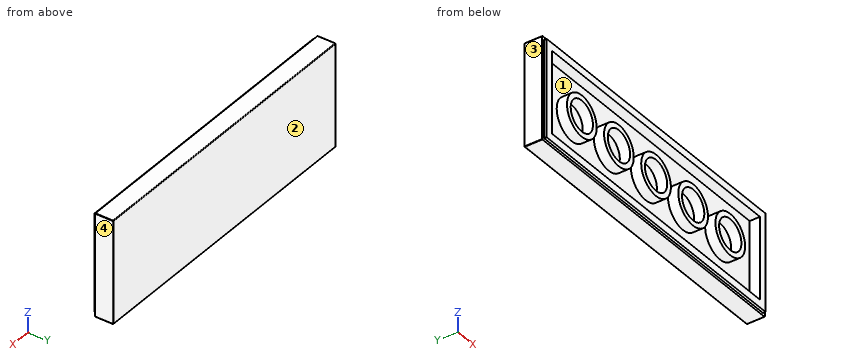
Autodesk Inventor part; units mm, degrees
ref_plane "YZ Plane" through (0, 0, 0) normal (1, 0, 0) x (0, 1, 0)
ref_plane "XZ Plane" through (0, 0, 0) normal (0, 1, 0) x (-1, 0, 0)
ref_plane "XY Plane" through (0, 0, 0) normal (0, 0, 1) x (1, 0, 0)
sketch "Sketch2" plane through (0, 0, 0) normal (0, 1, 0) x (-1, 0, 0)
  line L0 (-24, 8) -> (24, 8)
  line L1 (24, 8) -> (24, -8)
  line L2 (24, -8) -> (-24, -8)
  line L3 (-24, -8) -> (-24, 8)
  line L4 (-23.6, 7.6) -> (23.6, 7.6)
  line L5 (23.6, 7.6) -> (23.6, -7.6)
  line L6 (23.6, -7.6) -> (-23.6, -7.6)
  line L7 (-23.6, -7.6) -> (-23.6, 7.6)
  circle A0 centre (0, 0) radius 2.4
  circle A1 centre (0, 0) radius 3.2
  circle A2 centre (-8, 0) radius 2.4
  circle A3 centre (-8, 0) radius 3.2
  circle A4 centre (-16, 0) radius 2.4
  circle A5 centre (-16, 0) radius 3.2
  circle A6 centre (8, 0) radius 2.4
  circle A7 centre (8, 0) radius 3.2
  circle A8 centre (16, 0) radius 2.4
  circle A9 centre (16, 0) radius 3.2
  line L8 (16, 0) -> (8, 0) construction
  line L9 (8, 0) -> (0, 0) construction
  line L10 (0, 0) -> (-8, 0) construction
  line L11 (-8, 0) -> (-16, 0) construction
  line L12 (-22.4, 6.4) -> (22.4, 6.4)
  line L13 (22.4, 6.4) -> (22.4, -6.4)
  line L14 (22.4, -6.4) -> (-22.4, -6.4)
  line L15 (-22.4, -6.4) -> (-22.4, 6.4)
  circle A10 centre (-20, 4) radius 2.4 construction
  circle A11 centre (-20, -4) radius 2.4 construction
  circle A12 centre (20, 4) radius 2.4 construction
  circle A13 centre (20, -4) radius 2.4 construction
  point P0 (0, 8)
  point P1 (-24, 0)
  point P2 (0, 7.6)
  point P3 (-23.6, 0)
  point P4 (0, 6.4)
  point P5 (-22.4, 0)
  dimension "d0" = 16
  dimension "d1" = 48
  dimension "d2" = 0.4
  dimension "d3" = 0.4
  dimension "d4" = 4.8
  dimension "d5" = 6.4
  dimension "d6" = 8
  dimension "d7" = 1.6
  dimension "d8" = 1.6
  dimension "d15" = 4.8
extrude "Extrusion1" add sketch "Sketch2" along normal blind 3.2 contours L0 L1 L2 L3 | L4 L5 L6 L7 | A0 | A1 | A2 | A3 | A4 | A5 | A6 | A7 | A8 | A9 | L12 L13 L14 L15
extrude "Extrusion2" cut sketch "Sketch2" along normal blind 0.4 contours L0 L1 L2 L3
extrude "Extrusion3" cut sketch "Sketch2" along normal blind 1.6 contours A0 | A2 | A4 | A6 | A8 | L12 L13 L14 L15
fillet "Fillet1" radius 0.1 8 edges at (-24, 1.8, 8) (0, 3.2, 8) (-24, 3.2, 0) (-24, 1.8, -8) (0, 3.2, -8) (24, 1.8, -8) (24, 3.2, 0) (24, 1.8, 8)
sketch "Skizze3" plane through (0, 3.2, 0) normal (0, 1, 0) x (1, 0, 0)
  line L0 (23.9, 8) -> (-23.9, 8)
  line L1 (-24, 7.9) -> (-24, -7.9)
  line L2 (-23.9, -8) -> (23.9, -8)
  line L3 (23.9, -7.9) -> (-23.9, -7.9)
  line L4 (-24.9, -8.5) -> (-24.9, 8.1) construction
  line L5 (-24.9, 8.1) -> (28.7985, 8.1) construction
  line L6 (28.7985, 8.1) -> (28.7985, -8.5) construction
  line L7 (28.7985, -8.5) -> (-24.9, -8.5) construction
  point P0 (0, 0)
  dimension "d43" = 0.1
  dimension "d44" = 0.6
  dimension "d45" = 0.9
decal "Aufkleber1"
equation "\"d0\" = 2 * lu"
equation "\"d1\" = 6 * lu"
equation "\"d2\" = gw"
equation "\"d3\" = gw"
equation "\"d4\" = kd"
equation "\"d6\" = lu"
equation "\"d7\" = wall"
equation "\"d8\" = wall"
equation "\"d15\" = kd"
equation "\"d9\" = 0.333333 * lh"
equation "\"d11\" = gh"
equation "\"d13\" = 0.333333 * lh - topthk"
equation "\"d16\" = lf"
properties part number "42146_69729_2" material "ABS Plastic"
Could you check a few things on this model? Use its own coordinates, in mm. Face numbers are marked on the shaded views. Give positions to 0.01 mm unless a question says otherwise; leave off trailing zeros. Order: outer loops, then holes, each group sorted by start corner. A loop starts at its lowest first (then second) coordinate and runs counter-clockwise, first axis right, second up.
1. Thinking about a two-plate mould opening in X: for the marked faces 1, 2, 3 and 4, which applies, +X half, -X half, draft (parallel to the pull), parting line (faces both ways), or undercut?
Answers below:
face 1: undercut
face 2: draft
face 3: -X half
face 4: +X half
2. I need wall thicknesses on L1, parallel to Z at x = 8, y = 0.55; L2, parallel to Z at x = -14, y = 0.5; L3, parallel to Y at x = -19, z = -1.5. Which ranges of each line are inside material? Lowest first, please.
Answers below:
L1: z = -8 to -6.4, -3.2 to -2.4, 2.4 to 3.2, 6.4 to 8
L2: z = -8 to -6.4, -2.5 to -1.33, 1.33 to 2.5, 6.4 to 8
L3: y = 1.6 to 3.2
3. Suppose I cut it at C-C (z = 5). Write out the boundary of the cut face in (x, y).
Answers below:
outline: (-24, 0.4) - (-23.6, 0.4) - (-23.6, 0) - (-22.4, 0) - (-22.4, 1.6) - (22.4, 1.6) - (22.4, 0) - (23.6, 0) - (23.6, 0.4) - (24, 0.4) - (24, 3.1) arc R0.1 ccw to (23.9, 3.2) - (-23.9, 3.2) arc R0.1 ccw to (-24, 3.1) - close
4. For pin 1 (3 mm diameter, centred on x = -16, z = 0, fed in from -Y), with a flat end and sliding along its axis, tell me the tip position at first contact or that it passes through.
Answers below:
pin 1: stops at y = 1.6
5. Suppose I cut it at A-A (y = 1.1). State how many separate pieces and enclosed holes the cut face has, plus the area to 3 significant figures.
Answers below:
separate pieces: 6
enclosed holes: 6
area: 265 mm2
6. Suppose I cut it at B-B (x = -8). Write out the boundary of the cut face in (y, z), plus the area to 3 significant figures.
Answers below:
outline: (0, -7.6) - (0.4, -7.6) - (0.4, -8) - (3.1, -8) arc R0.1 ccw to (3.2, -7.9) - (3.2, 7.9) arc R0.1 ccw to (3.1, 8) - (0.4, 8) - (0.4, 7.6) - (0, 7.6) - (0, 6.4) - (1.6, 6.4) - (1.6, 3.2) - (0, 3.2) - (0, 2.4) - (1.6, 2.4) - (1.6, -2.4) - (0, -2.4) - (0, -3.2) - (1.6, -3.2) - (1.6, -6.4) - (0, -6.4) - close
area: 33.0 mm2
7. Suppose I cut it at D-D (x = 12). Write out the boundary of the cut face in (y, z), plus the area to 3 significant figures.
Answers below:
outline: (0, -7.6) - (0.4, -7.6) - (0.4, -8) - (3.1, -8) arc R0.1 ccw to (3.2, -7.9) - (3.2, 7.9) arc R0.1 ccw to (3.1, 8) - (0.4, 8) - (0.4, 7.6) - (0, 7.6) - (0, 6.4) - (1.6, 6.4) - (1.6, -6.4) - (0, -6.4) - close
area: 30.4 mm2
